Model file for the job. Use its own axes, mm. A direction names the side the tool comes from. Coordinates: 2 decimals unless noted, no trailing zeros. Write each loop counter-clockwise with the first axis right and the second up, starting at its lowest first coordinate (ties: lowest second). Pieces come first, ordered by that corner, then holes. Notation, with made-up numbers: M -5,-32.75 L 37,-32.75 A12 ccw 37,-13.75 Z; hole C 83.5,16 d3. An arc over 180 degrees is marked long. Use CSV: the item, a comma, the result in double quotes. Start each with the question number.
from build123d import *

# Parameters (mm, degrees)
BOSS_EXTRUDE1_DEPTH      = 34
SKETCH2_R                = 3.503672553
BOSS_EXTRUDE2_DEPTH      = 3
SKETCH3_R                = 1.746279777
BOSS_EXTRUDE3_DEPTH      = 3
SKETCH4_R                = 0.749347306
BOSS_EXTRUDE4_DEPTH      = 6
SKETCH5_W                = 4
SKETCH5_H                = 42.204508387
BOSS_EXTRUDE5_DEPTH      = 3
BOSS_EXTRUDE7_DEPTH      = 0.5
BOSS_EXTRUDE7_DEPTH_BACK = 0.5
SKETCH7_W                = 36.186676628
SKETCH7_H                = 9.506502519


with BuildPart() as part:
    # Sketch1 → Boss-Extrude1 (new body)
    with BuildSketch(Plane.XY):
        with BuildLine():
            Line((-11.599484275, 16.292696663), (11.599484275, 16.292696663))
            ThreePointArc((11.599484275, 16.292696663), (20, 0), (11.599484275, -16.292696663))
            Line((11.599484275, -16.292696663), (-11.599484275, -16.292696663))
            ThreePointArc((-11.599484275, -16.292696663), (-20, 0), (-11.599484275, 16.292696663))
        make_face()
    extrude(amount=BOSS_EXTRUDE1_DEPTH)

    # Sketch2 → Boss-Extrude2 (add)
    with BuildSketch(Plane.XY.offset(34)):
        Circle(SKETCH2_R)
    extrude(amount=BOSS_EXTRUDE2_DEPTH)

    # Sketch3 → Boss-Extrude3 (add)
    with BuildSketch(Plane.XY.offset(37)):
        Circle(SKETCH3_R)
    extrude(amount=BOSS_EXTRUDE3_DEPTH)

    # Sketch4 → Boss-Extrude4 (add)
    with BuildSketch(Plane.XY.offset(40)):
        Circle(SKETCH4_R)
    extrude(amount=BOSS_EXTRUDE4_DEPTH)

    # Sketch5 → Boss-Extrude5 (add)
    with BuildSketch(Plane(origin=(0, 0, 0), x_dir=(-1, 0, 0), z_dir=(0, 0, -1))):
        with Locations((-8.261138403, 0.267681872)):
            Rectangle(SKETCH5_W, SKETCH5_H)
        with Locations((7.442864718, 0.267681872)):
            Rectangle(SKETCH5_W, SKETCH5_H)
    extrude(amount=BOSS_EXTRUDE5_DEPTH)

    # Sketch7 → Boss-Extrude7 (add, two sides: drawn at the far end of the back side and taken through both)
    with BuildSketch(Plane(origin=(0, 0, 0), x_dir=(1, 0, 0), z_dir=(0, 1, 0)).offset(-BOSS_EXTRUDE7_DEPTH_BACK)):
        with Locations((0.761824771, -45.603600446)):
            Rectangle(SKETCH7_W, SKETCH7_H)
    extrude(amount=BOSS_EXTRUDE7_DEPTH + BOSS_EXTRUDE7_DEPTH_BACK)


solid = part.part
1) Wall check: L1, parallel to Z at x = 16, y = -4; L2, parallel to Y at x = -8.5, z = 3.5; L3, parallel to Y at x = 10.5, z = 48.5. Give the ranges that are in metal, low to high. Write a range as [from, to].
2) Band-saw the part on C-C on z = 6. List the corners of the cut face in (x, y), then the cut area to 3 significant figures.
3) Drop flat-ended pins along their axis: P1, Ø9.5, axis at x = -2, y = -6.5, coming from the -Z side; P2, Ø4, axis at x = 4.5, z = 44.5, coming from the -Y side; P3, Ø1, axis at x = -14, z = 35, coming from the +Y side; P4, Ø3, axis at x = 8.5, y = 19.5, coming from the +Z side. Give the stop position or say it passes through.
4) Band-saw the part on D-D on x = 8.5. List the corners of the cut face in (y, z).
5) Tool access for faces 5 (the face through (-7, -19, 0)), 6 (the face through (0, 16.293, 17)), 7 (the face through (6.261, 0, -1)): list every direction of +Z, -Z, +X, -X, +Y, -Y with a clear straight run to the whole face (end or side of a thin tool).
6) Band-saw the part on A-A on x = 17. List the corners of the cut face in (y, z), then the cut area to 3 significant figures.
7) Two-plate mould, pull along Z, no slides. Class faces 1 (the face through (0, -1, 40)), 2 (the face through (8, 19, 0)), 3 (the face through (10.261, 0, -1)), 4 (the face through (-13, 0, 0)): pulls with the +Z half, pulls with the -Z half, needs draft (parallel to the pull), parting line crosses it, or undercut.
8) Band-saw the part on B-B on y = -11.5. List the corners of the cut face in (x, z).
Findings below:
1,L1,"z = [0, 34]"
1,L2,"y = [-16.29, 16.29]"
1,L3,"y = [-0.5, 0.5]"
2,outline,"M -11.6,-16.29 L 11.6,-16.29 A20 ccw 11.6,16.29 L -11.6,16.29 A20 ccw Z"
2,area,"1,140 mm2"
3,P1,"stops at z = -3"
3,P2,"stops at y = -0.5"
3,P3,"passes through"
3,P4,"stops at z = 0"
4,outline,"M -20.83,-3 L 21.37,-3 L 21.37,0 L 16.29,0 L 16.29,34 L -16.29,34 L -16.29,0 L -20.83,0 Z; M -0.5,40.85 L 0.5,40.85 L 0.5,50.36 L -0.5,50.36 Z"
5,face 5,"+Z, +X, -X, -Y"
5,face 6,"+Z, +X, -X, +Y"
5,face 7,"-Z, +Y, -Y"
6,outline,"M -10.54,0 L 10.54,0 L 10.54,34 L -10.54,34 Z; M -0.5,40.85 L 0.5,40.85 L 0.5,50.36 L -0.5,50.36 Z"
6,area,"726 mm2"
7,face 1,"undercut"
7,face 2,"pulls with the +Z half"
7,face 3,"needs draft"
7,face 4,"pulls with the -Z half"
8,outline,"M -16.36,0 L -9.44,0 L -9.44,-3 L -5.44,-3 L -5.44,0 L 6.26,0 L 6.26,-3 L 10.26,-3 L 10.26,0 L 16.36,0 L 16.36,34 L -16.36,34 Z"
